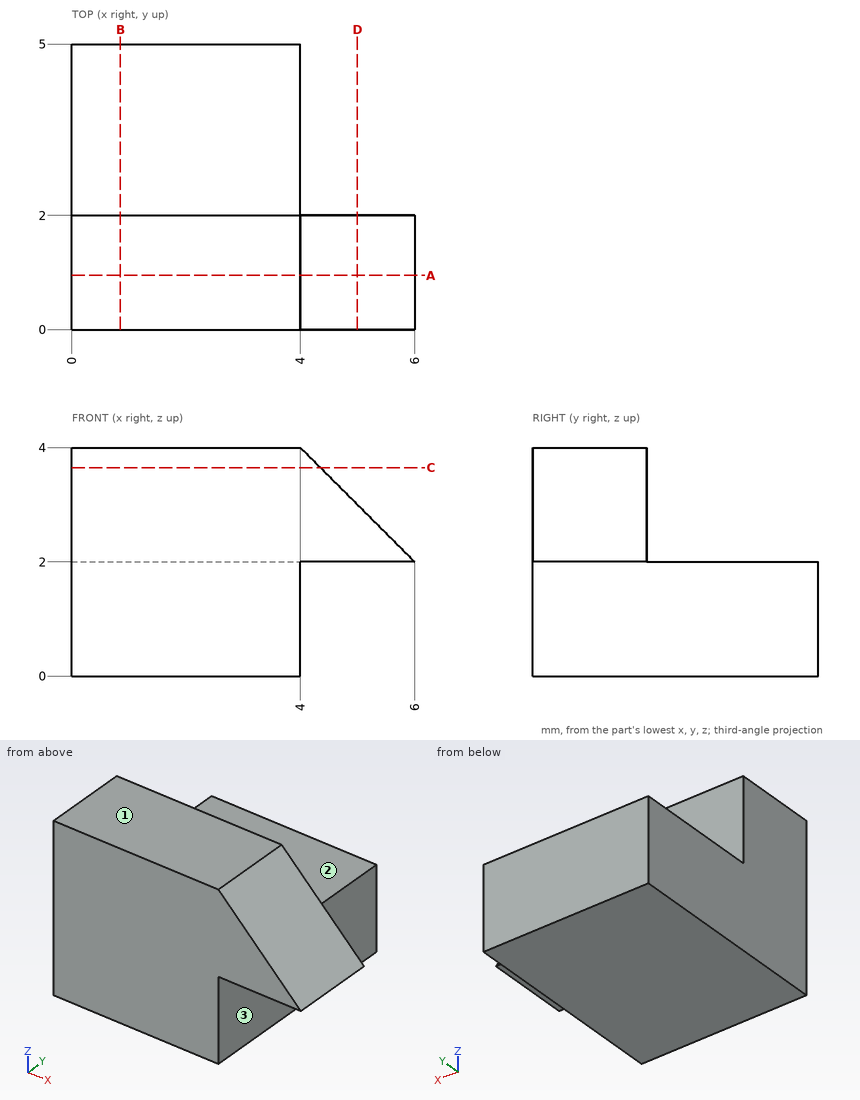
The drawing under review shows one solid part. Ordinate dimensions are in mm from its lowest x, y, z. A direction names the side the tool comes from. Round coordinates to 2 decimals unless told otherwise and drop trailing zeros. Loops run counter-clockwise (first coordinate to the right, second up) from the corner with the lowest first, then second, coordinate; pieces in that order, holes last. Notation, with made-up numbers: (59, -16.5) - (106, -16.5) arc R16 cw to (106, 0.5) - close; hole circle Ø7 at (65, 80). An arc over 180 degrees is marked (long way). One line per question, with ' | ' between items.
Q1. Take a section at A-A (y = 0.95). Give the boundary of the cut face in (x, z).
Taken from the geometry:
outline: (0, 0) - (4, 0) - (4, 2) - (6, 2) - (4, 4) - (0, 4) - close
Q2. Take a section at C-C (z = 3.65). Give the boundary of the cut face in (x, y).
Taken from the geometry:
outline: (0, 0) - (4.35, 0) - (4.35, 2) - (0, 2) - close
Q3. Take a section at D-D (x = 5). Give the boundary of the cut face in (y, z), and give its area (3 significant figures).
Taken from the geometry:
outline: (0, 2) - (2, 2) - (2, 3) - (0, 3) - close | area: 2.00 mm²
Q4. For pin 1 (1.5 mm diameter, centred on x = 5.5, y = 1.5, fed in from -Z); pin 2 (0.6 mm diameter, centred on x = 2, z = 3, fed in from +Y); pin 3 (1 mm diameter, centred on y = 1.5, z = 1, fed in from +X), all flat-tipped, find the tip position at first contact; note any pin that passes through.
Taken from the geometry:
pin 1: stops at z = 2 | pin 2: stops at y = 2 | pin 3: stops at x = 4
Q5. For line 1 along X through (y, z) = (1.45, 0.45); line 2 along Y through (x, z) = (0.8, 3.45), list the stretches that pass through material, from the lowest coordinate up. Write a range as [from, to].
Taken from the geometry:
line 1: x = [0, 4] | line 2: y = [0, 2]
Q6. Tool access review of the marked faces 1, 2 and 3: name each direction out of +Z, -Z, +X, -X, +Y, -Y from which nothing blocks a thin tool from reaching the whole face with its end or side.
Taken from the geometry:
face 1: +Z, +X, -X, +Y, -Y | face 2: +Z, +X, -X, +Y | face 3: -Z, +X, +Y, -Y
Q7. Take a section at B-B (x = 0.85). Give the boundary of the cut face in (y, z), and give its area (3 significant figures).
Taken from the geometry:
outline: (0, 0) - (5, 0) - (5, 2) - (2, 2) - (2, 4) - (0, 4) - close | area: 14.0 mm²
